```python
from build123d import *

# Parameters (mm, degrees)
SKETCH_1_W          = 45.3
SKETCH_1_H          = 20.5
SKETCH_1_R          = 8
SKETCH_1_R_2        = 1
EXTRUDE_1_DEPTH     = 1.2
EXTRUDE_START       = -1.2
SKETCH_2_R          = 8
EXTRUDE_2_DEPTH     = 13.3
SKETCH_3_W          = 8
SKETCH_3_H          = 3
EXTRUDE_3_DEPTH     = 4.8
SKETCH_5_W          = 7.748347941
SKETCH_5_H          = 3.984864655
SKETCH_5_W_2        = 9.563675173
SKETCH_5_H_2        = 6.597164818
SKETCH_5_W_3        = 5.313152873
SKETCH_5_H_3        = 11.201897308
EXTRUDE_4_DEPTH     = 3
CUT_EXTRUDE_1_REACH = 30.195
SKETCH_6_R          = 1.27


with BuildPart() as part:
    # 草图1 → 凸台-拉伸1 (new body)
    with BuildSketch(Plane.XY):
        Rectangle(SKETCH_1_W, SKETCH_1_H)
        with Locations((-13, 0)):
            Circle(SKETCH_1_R, mode=Mode.SUBTRACT)
        with Locations((13, 0)):
            Circle(SKETCH_1_R, mode=Mode.SUBTRACT)
        with Locations((-21.15, 8.75)):
            Circle(SKETCH_1_R_2, mode=Mode.SUBTRACT)
        with Locations(Location((21.15, 8.75, 0), (0, 0, 180))):
            Circle(SKETCH_1_R_2, mode=Mode.SUBTRACT)
        with Locations(Location((-21.15, -8.75, 0), (0, 0, 180))):
            Circle(SKETCH_1_R_2, mode=Mode.SUBTRACT)
        with Locations((21.15, -8.75)):
            Circle(SKETCH_1_R_2, mode=Mode.SUBTRACT)
    extrude(amount=EXTRUDE_1_DEPTH)

    # 草图2 → 凸台-拉伸2 (add)
    with BuildSketch(Plane.XY.offset(1.2).offset(EXTRUDE_START)):
        with Locations((13, 0)):
            Circle(SKETCH_2_R)
        with Locations((-13, 0)):
            Circle(SKETCH_2_R)
    extrude(amount=EXTRUDE_2_DEPTH)

    # 草图3 → 凸台-拉伸3 (add)
    with BuildSketch(Plane.XY.offset(1.2).offset(EXTRUDE_START)):
        with Locations((0, 7.75)):
            Rectangle(SKETCH_3_W, SKETCH_3_H)
    extrude(amount=EXTRUDE_3_DEPTH)

    # 草图5 → 凸台-拉伸4 (add)
    with BuildSketch(Plane(origin=(0, 0, 0), x_dir=(-1, 0, 0), z_dir=(0, 0, -1)).offset(EXTRUDE_START)):
        with Locations((-18.131134181, -0.464900877)):
            Rectangle(SKETCH_5_W, SKETCH_5_H)
        with Locations((-0.398486465, 0.841249205)):
            Rectangle(SKETCH_5_W_2, SKETCH_5_H_2)
        with Locations((18.950245248, 0.309933918)):
            Rectangle(SKETCH_5_W_3, SKETCH_5_H_3)
    extrude(amount=EXTRUDE_4_DEPTH)

    # 草图6 → 切除-拉伸1 (cut, up to next)
    with BuildSketch(Plane(origin=(0, 0, 0), x_dir=(-1, 0, 0), z_dir=(0, 0, -1)), mode=Mode.PRIVATE) as cut_extrude_1_sk1:
        with Locations((-4.031891603, -8.25)):
            Circle(SKETCH_6_R)
    cut_extrude_1_tool1 = extrude(cut_extrude_1_sk1.sketch, amount=-CUT_EXTRUDE_1_REACH, mode=Mode.PRIVATE) & part.part
    add(cut_extrude_1_tool1.solids().sort_by_distance((4.031892, -8.25, 0))[0], mode=Mode.SUBTRACT)


solid = part.part
```
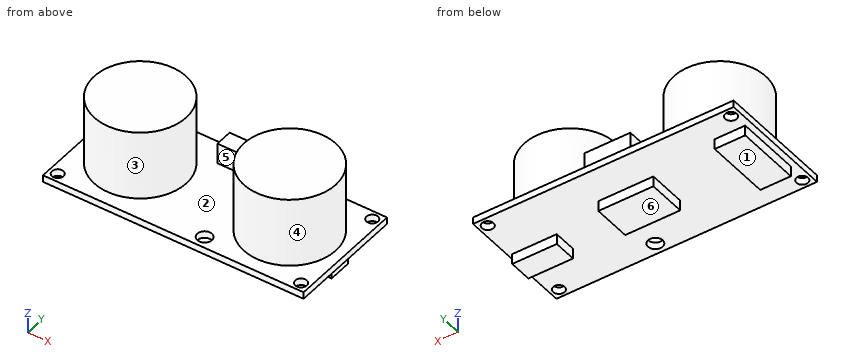
Build history of the part. All positions in model axes, mm. Face numbers are marked on the shaded views. A direction names the side the tool comes from. Give positions to 0.01 mm unless a question says otherwise; leave off trailing zeros. Loops run counter-clockwise (first coordinate to the right, second up) from the corner with the lowest first, then second, coordinate; pieces in that order, holes last.
1) Band-saw the part on B-B on y = -8.75. List the corners of the cut face in (x, z), then the cut area to 3 significant figures.
Values follow:
outline: (-22.65, 0) - (-22.15, 0) - (-22.15, 1.2) - (-22.65, 1.2) - close; (-20.15, 0) - (2.86, 0) - (2.86, 1.2) - (-20.15, 1.2) - close; (5.2, 0) - (20.15, 0) - (20.15, 1.2) - (5.2, 1.2) - close; (22.15, 0) - (22.65, 0) - (22.65, 1.2) - (22.15, 1.2) - close
area: 46.8 mm2
2) Band-saw the part on C-C on x = -0.5. List the corners of the cut face in (y, z), then the cut area to 3 significant figures.
Values follow:
outline: (-10.25, 0) - (-2.46, 0) - (-2.46, -1.8) - (4.14, -1.8) - (4.14, 0) - (10.25, 0) - (10.25, 1.2) - (9.25, 1.2) - (9.25, 4.8) - (6.25, 4.8) - (6.25, 1.2) - (-10.25, 1.2) - close
area: 47.3 mm2
3) 3-axis set-ups, long thin cutter, end or side, ignore diameter. For the marked faces 4, 5 and 6: which of +Z, -Z, +X, -X, +Y, -Y reach the whole face in a straight line?
Values follow:
face 4: +Z
face 5: +Z, -Y
face 6: -Z, +X, -X, +Y, -Y
4) Two-plate mould, pull along X, no slides. Class the marked faces 1, 2 and 3: released by +X, released by -X, zero draft, split by the parting line, or undercut.
Values follow:
face 1: zero draft
face 2: undercut
face 3: undercut
5) Band-saw the part on D-D on z = 0.5. List the corners of the cut face in (x, y).
Values follow:
outline: (-22.65, -10.25) - (22.65, -10.25) - (22.65, 10.25) - (-22.65, 10.25) - close; hole circle Ø2 at (-21.15, -8.75); hole circle Ø2 at (-21.15, 8.75); hole circle Ø2.54 at (4.03, -8.25); hole circle Ø2 at (21.15, -8.75); hole circle Ø2 at (21.15, 8.75)
6) Drop flat-ended pins along their axis: P1, Ø1.2, axis at x = 21.15, y = -8.75, coming from the +Z side; P2, Ø4, axis at x = 12.5, z = 5.5, coming from the +Y side; P3, Ø2, axis at x = -18, z = -1.5, coming from the -Y side; P4, Ø2, axis at x = 1, y = 7, coming from the -Z side. Give the stop position or say it passes through.
Values follow:
P1: passes through
P2: stops at y = 8
P3: stops at y = -5.29
P4: stops at z = 0
7) Probe line 1 along Y through (x, z) = (-21.15, 0.5); line 2 along X through (y, z) = (3, -1); line 3 along Z through (x, y) = (-7.5, -9.5). List the from-to ranges inside material, lowest first.
Values follow:
line 1: y = -10.25 to -9.75, -7.75 to 7.75, 9.75 to 10.25
line 2: x = -21.61 to -16.29, -4.38 to 5.18
line 3: z = 0 to 1.2
8) Band-saw the part on A-A on z = 3. List the corners of the cut face in (x, y).
Values follow:
outline: circle Ø16 at (-13, 0); (-4, 6.25) - (4, 6.25) - (4, 9.25) - (-4, 9.25) - close; circle Ø16 at (13, 0)
